For this review, take the finished solid that the model builds, in its own axes (mm). Give positions to 0.01 mm unless a question says otherwise; leave off trailing zeros. Loops run counter-clockwise (first coordinate to the right, second up) from the corner with the lowest first, then second, coordinate; pieces in that order, holes last. Notation, with made-up numbers: (56, 86) - (99, 86) arc R6 cw to (99, 94) - close; hole circle Ø2 at (55.25, 40.25). An arc over 180 degrees is marked (long way). Answer in a Markdown table with one row per item.
```python
from build123d import *

# Parameters (mm, degrees)
SKETCH034_R     = 3.925
SKETCH034_R_2   = 1.75
PAD016_DEPTH    = 1.5
SKETCH035_R     = 3.925
PAD017_DEPTH    = 2
CHAMFER001_SIZE = 0.3


with BuildPart() as part:
    # Sketch034 (on DatumPlane) → Pad016 (new body)
    with BuildSketch(Plane(origin=(0.0002244487, 33.0000455142, 5.0001576066), x_dir=(-0.999999999, 4e-10, 4.48856e-05), z_dir=(0, -1, 9.1023e-06))):
        with Locations((27.900008, 3)):
            Circle(SKETCH034_R)
        with Locations((27.900008, 3)):
            Circle(SKETCH034_R_2, mode=Mode.SUBTRACT)
    extrude(amount=PAD016_DEPTH)

    # Sketch035 (on Face4 of Pad016) → Pad017 (join)
    with BuildSketch(Plane(origin=(0.0002244487, 31.5000455143, 5.00017126), x_dir=(-0.999999999, 4e-10, 4.48856e-05), z_dir=(0, -1, 9.1023e-06))):
        with Locations((27.900008, 3)):
            Circle(SKETCH035_R)
    extrude(amount=PAD017_DEPTH)

    # Chamfer001
    chamfer001_edges = [part.edges().sort_by_distance(p)[0] for p in [
        (-26.149918, 33.000018, 2.001331),
    ]]
    chamfer(chamfer001_edges, length=CHAMFER001_SIZE)


solid = part.part
```
1. Clearance check with flat-ended pins moving along their axes: pin 1 (1 mm diameter, centred on x = -28, z = 1.5, fed in from +Y); pin 2 (1.5 mm diameter, centred on x = -27, y = 32.5, fed in from -Z). State where each tip first meets the part, or that it passes through.
Values:
| item | result |
|---|---|
| pin 1 | stops at y = 31.5 |
| pin 2 | stops at z = -1.92 |
2. We need section B-B, the plane x = -30.75. Give the boundary of the cut face in (y, z).
Values:
| item | result |
|---|---|
| outline | (29.5, -0.7) - (33, -0.7) - (33, 4.7) - (29.5, 4.7) - close |
3. Mouldability with a two-part tool opening along X and no side actions: class faces 1 (the face through (-31.526, 31.275, 3.505)), 2 (the face through (-26.15, 32.11, 1.92)) as released by +X, released by -X, zero draft, split by the parting line, or undercut.
Values:
| item | result |
|---|---|
| face 1 | split by the parting line |
| face 2 | undercut |
4. Wall thickness on line 1 (Y direction, x = -28, z = 2.5); line 2 (X direction, y = 31.8, z = 1.5); line 3 (X direction, y = 32.4, z = 3.5): over which ranges is each line inside the solid? List them lowest first. Write a range as [from, to].
Values:
| item | result |
|---|---|
| line 1 | y = [29.5, 31.5] |
| line 2 | x = [-31.79, -29.58], [-26.22, -24.01] |
| line 3 | x = [-31.53, -28.8], [-27, -24.27] |
5. We need section A-A, the plane x = -25.5. Give the boundary of the cut face in (y, z).
Values:
| item | result |
|---|---|
| outline | (29.5, -1.1) - (33, -1.1) - (33, 5.11) - (29.5, 5.11) - close |
